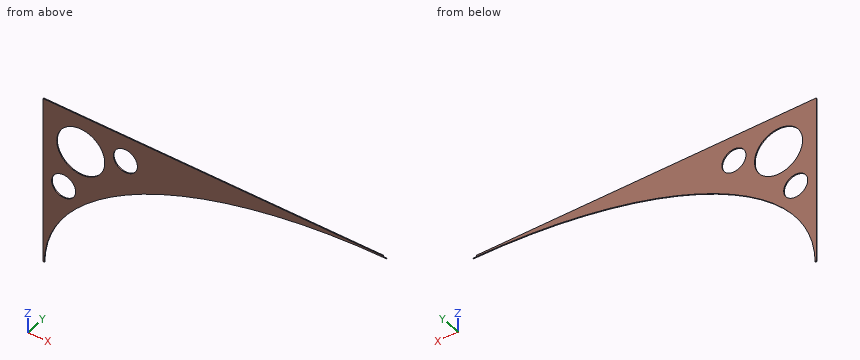
from build123d import *

# Parameters (mm, degrees)
F1_DEPTH = 1.4
F3_D     = 70
F4_D     = 35
F5_W     = 5
F5_H     = 1.4
F6_DEPTH = 2


with BuildPart() as f1:
    # F0 (on Front) → F1 (new body)
    with BuildSketch(Plane.XZ):
        with BuildLine():
            Line((234.3109268695, 164.7265180945), (-265.6890731305, 164.7265180945))
            Line((-265.6890731305, 164.7265180945), (-265.6890731305, -85.2734819055))
            Line((-265.6890731305, -85.2734819055), (-263.6890731305, -85.2734819055))
            add(Edge.make_bspline(
                [(234.3109268695, 162.7265180945), (-263.6890731305, 162.7265180945), (-263.6890731305, -85.2734819055)],
                knots=[4.7123889804, 4.7123889804, 4.7123889804, 6.2831853072, 6.2831853072, 6.2831853072], degree=2, weights=[1, 0.7071067812, 1]))
            Line((234.3109268695, 162.7265180945), (234.3109268695, 164.7265180945))
        make_face()
    extrude(amount=F1_DEPTH)

    # F3 (through all)
    with Locations(Plane.XZ.offset(1.4)):
        with Locations((-210.6890731305, 109.7265180945)):
            Hole(F3_D / 2)

    # F4 (through all)
    with Locations(Plane.XZ.offset(1.4)):
        with Locations((-145.6890731305, 127.2265180945), (-235.6890731305, 44.7265180945)):
            Hole(F4_D / 2)

    # F5 (on face) → F6 (cut)
    with BuildSketch(Plane.XY.offset(164.7265180945)):
        Polygon((239.3109268695, -5.7), (239.3109268695, 4.3), (229.3109268695, 4.3), (229.3109268695, 0), (234.3109268695, 0), (234.3109268695, -1.4), (229.3109268695, -1.4), (229.3109268695, -5.7), align=None)
        with Locations((231.8109268695, -0.7)):
            Rectangle(F5_W, F5_H)
    extrude(amount=-F6_DEPTH, mode=Mode.SUBTRACT)


solid = f1.part
Input: part model. Units: mm. Frame: model coordinates. Coordinates: 2 decimals unless noted, no trailing zeros.
Q1. Material intervals for line 1 (Z direction, x = -237, y = -0.95); line 2 (Z direction, x = -243, y = -0.7); line 3 (Z direction, x = -194.5, y = -0.75), sorted ascending.
Q2. Contact query for a flat-ended pin moving along its axis: pin 1 (5 mm diameter, centred on x = -186, z = 134, fed in from +Y). Output: stop coordinate, or through.
Q3. Cut plane A-A (z = 122.5). Give the number of separate pieces and of enclosed holes in the cut face, then the cut area to 3 significant figures.
Working result:
1. line 1: z = -5.18 to 27.28, 62.18 to 86.65, 132.81 to 164.73
1. line 2: z = -14.53 to 28.83, 60.63 to 96.27, 123.18 to 164.73
1. line 3: z = 40.83 to 78.7, 140.76 to 164.73
2. pin 1: stops at y = 0
3. separate pieces: 3
3. enclosed holes: 0
3. area: 181 mm2
